Here's how the part is built. I have some questions about the finished solid (model axes, mm). A direction names the side the tool comes from. Round coordinates to 2 decimals unless told otherwise and drop trailing zeros. Order: outer loops, then holes, each group sorted by start corner. A loop starts at its lowest first (then second) coordinate and runs counter-clockwise, first axis right, second up.
```python
from build123d import *

# Parameters (mm, degrees)
SKETCH1_R             = 16
SKETCH1_R_2           = 4
SKETCH1_R_3           = 2
BOSS_EXTRUDE1_DEPTH   = 3
SKETCH2_R             = 8
SKETCH2_R_2           = 4
BOSS_EXTRUDE2_DEPTH   = 13
BODY_MOVE_COPY1_ANGLE = 90


with BuildPart() as part:
    # Sketch1 → Boss-Extrude1 (new body)
    with BuildSketch(Plane(origin=(0, 0, 0), x_dir=(1, 0, 0), z_dir=(0, 1, 0))):
        Circle(SKETCH1_R)
        Circle(SKETCH1_R_2, mode=Mode.SUBTRACT)
        with Locations((12, 0)):
            Circle(SKETCH1_R_3, mode=Mode.SUBTRACT)
        with Locations((0, -12)):
            Circle(SKETCH1_R_3, mode=Mode.SUBTRACT)
        with Locations((-12, 0)):
            Circle(SKETCH1_R_3, mode=Mode.SUBTRACT)
        with Locations((0, 12)):
            Circle(SKETCH1_R_3, mode=Mode.SUBTRACT)
    extrude(amount=BOSS_EXTRUDE1_DEPTH)

    # Sketch2 → Boss-Extrude2 (add)
    with BuildSketch(Plane(origin=(0, 0, 0), x_dir=(1, 0, 0), z_dir=(0, 1, 0))):
        Circle(SKETCH2_R)
        Circle(SKETCH2_R_2, mode=Mode.SUBTRACT)
    extrude(amount=BOSS_EXTRUDE2_DEPTH)


with BuildPart() as part_1:
    # Body-Move/Copy1: moved
    add(part.part.rotate(Axis((0, 6.5, 0), (-1, 0, 0)), BODY_MOVE_COPY1_ANGLE))


solid = part_1.part
```
1) For faces 1 (the cylindrical face through (-0.867, 10.405, 0.091)), 2 (the flat face through (-4, -1, 3.5)), which set-ups out of +Z, -Z, +X, -X, +Y, -Y let a thin tool reach every point of the face, with its end or its side?
2) If we section it at A-A (x = 0): Write out the boundary of the cut face in (y, z).
3) If we section it at B-B (y = 6.5): Write out the boundary of the cut face in (x, z).
4) If we section it at D-D (y = -6.5): Write out the boundary of the cut face in (x, z).
5) I'm going to push flat-ended pins straight in: pin 1 (2 mm diameter, centred on x = -6, z = -1.5, fed in from -Y) (3 decimals); pin 2 (6 mm diameter, centred on y = -3.5, z = 4.5, fed in from +X); pin 3 (4 mm diameter, centred on y = 17.5, z = 5, fed in from -X). Where does each tip first touch, or does it pass through?
6) We'd pull the mould along X, two halves only. Please class faces 3 (the cylindrical face through (-0.26, -7.483, 5.021)), 4 (the cylindrical face through (10.002, 6.412, 5.021)), 5 (the flat face through (3, 10, 6.5)), 6 (the cylindrical face through (-1.73, 14.31, -1.43)): +X half, -X half, draft (parallel to the pull), parting line (faces both ways), or undercut.
7) If we section it at C-C (z = 5.25): Write out the boundary of the cut face in (x, y).
8) I need wall thicknesses on line 1 (Y direction, x = 0, z = 5.2); line 2 (X direction, y = 6.5, z = 5.85); line 3 (Y direction, x = 0, z = -0.5). Which ranges of each line are inside material? Lowest first, please.
Solutions:
1. face 1: +Z, -Z
1. face 2: -Z
2. outline: (-9.5, 3.5) - (-7.5, 3.5) - (-7.5, 6.5) - (-9.5, 6.5) - close; (-3.5, 3.5) - (-1.5, 3.5) - (-1.5, -6.5) - (2.5, -6.5) - (2.5, 6.5) - (-3.5, 6.5) - close; (10.5, -6.5) - (14.5, -6.5) - (14.5, 3.5) - (16.5, 3.5) - (16.5, 6.5) - (10.5, 6.5) - close; (20.5, 3.5) - (22.5, 3.5) - (22.5, 6.5) - (20.5, 6.5) - close
3. outline: (-16, 3.5) - (-14, 3.5) - (-14, 6.5) - (-16, 6.5) - close; (-10, 3.5) - (-8, 3.5) - (-8, -6.5) - (-4, -6.5) - (-4, 6.5) - (-10, 6.5) - close; (4, -6.5) - (8, -6.5) - (8, 3.5) - (10, 3.5) - (10, 6.5) - (4, 6.5) - close; (14, 3.5) - (16, 3.5) - (16, 6.5) - (14, 6.5) - close
4. outline: (-9.33, 3.5) - (-1.73, 3.5) - (-1.73, 6.5) - (-9.33, 6.5) - close; (1.73, 3.5) - (9.33, 3.5) - (9.33, 6.5) - (1.73, 6.5) - close
5. pin 1: stops at y = 0.255
5. pin 2: stops at x = 14.39
5. pin 3: stops at x = -13.23
6. face 3: undercut
6. face 4: undercut
6. face 5: draft
6. face 6: parting line
7. outline: circle Ø32 at (0, 6.5); hole circle Ø4 at (-12, 6.5); hole circle Ø8 at (0, 6.5); hole circle Ø4 at (0, -5.5); hole circle Ø4 at (0, 18.5); hole circle Ø4 at (12, 6.5)
8. line 1: y = -9.5 to -7.5, -3.5 to 2.5, 10.5 to 16.5, 20.5 to 22.5
8. line 2: x = -16 to -14, -10 to -4, 4 to 10, 14 to 16
8. line 3: y = -1.5 to 2.5, 10.5 to 14.5
